Study the drawing (mm; zero at the part's minimum x, y, z) and answer. A direction names the side the tool comes from. Give positions to 0.01 mm unless a question says otherwise; leave off trailing zeros. Order: outer loops, then holes, each group sorted by start corner. A loop starts at its lowest first (then second) coordinate and runs counter-clockwise, first axis right, second up. Notation, with made-up numbers: (-32.5, -5.75) -> (24.5, -5.75) arc R16 cw to (24.5, 2.25) -> close; hole circle Ø11 at (23, 53.5). An arc over 180 degrees is marked (long way). Use a Markdown table: item, result. Add a question column.
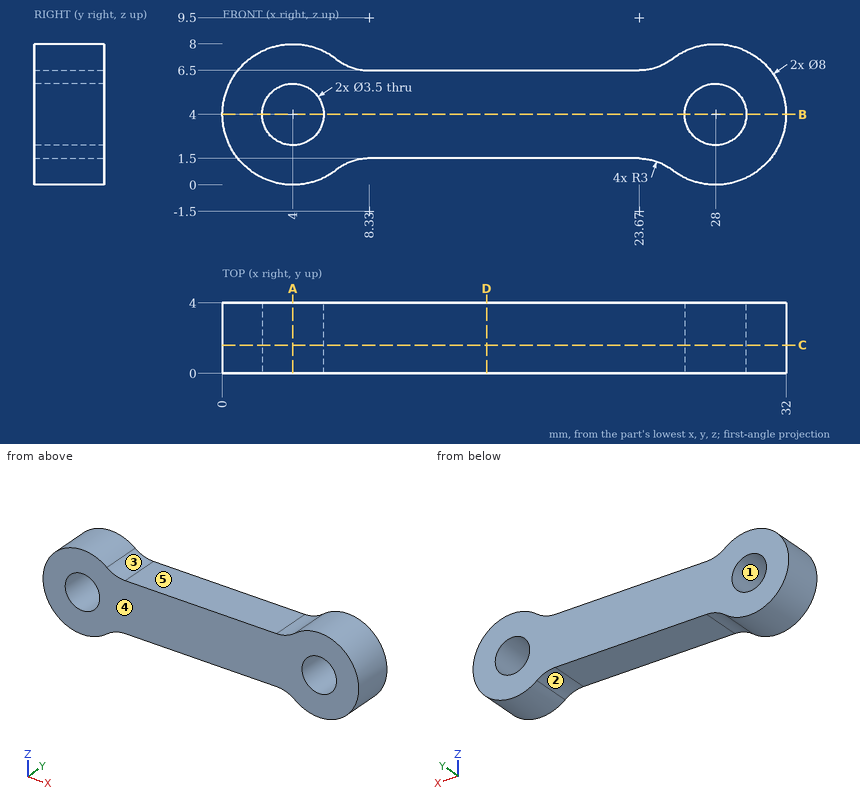
1) The part is cut by section A-A, the plane x = 4. Determine the outline of the cut face in (y, z).
2) Flat-ended cylindrical pins translate along their axes: pin 1 (2 mm diameter, centred on x = 16, y = 3, fed in from -Z); pin 2 (4.5 mm diameter, centred on x = 4, z = 4, fed in from +Y). Find the tip coordinate at first contact, or state that the pin passes through.
3) Which of the six approach directions +Z, -Z, +X, -X, +Y, -Y give full straight-line access (tool end or side, diameter ignored) to the marked faces 1, 2 and 3?
4) Determine the mould class of the marked faces 4 and 5 for opening direction X: released by +X, released by -X, zero draft, split by the parting line, or undercut.
5) The part is cut by section C-C, the plane y = 1.6. Determine the outline of the cut face in (x, z).
6) The part is cut by section B-B, the plane z = 4. Determine the outline of the cut face in (x, y), then the cut area to 3 significant figures.
7) Straight lines are drawn through the part: line 1 (X direction, y = 2, z = 4); line 2 (X direction, y = 3.4, z = 5); line 3 (Z direction, x = 4, y = 2.9). For each, find the intervals that lie inside material, in ascending order.
8) The part is cut by section D-D, the plane x = 15. Determine the outline of the cut face in (y, z), then the cut area to 3 significant figures.
A:
| question | item | result |
|---|---|---|
| 1 | outline | (0, 0) -> (4, 0) -> (4, 2.25) -> (0, 2.25) -> close; (0, 5.75) -> (4, 5.75) -> (4, 8) -> (0, 8) -> close |
| 2 | pin 1 | z = 1.5 |
| 2 | pin 2 | y = 4 |
| 3 | face 1 | +Y, -Y |
| 3 | face 2 | -Z, +Y, -Y |
| 3 | face 3 | +Z, +Y, -Y |
| 4 | face 4 | zero draft |
| 4 | face 5 | undercut |
| 5 | outline | (6.47, 0.86) arc R3 cw to (8.33, 1.5) -> (23.67, 1.5) arc R3 cw to (25.53, 0.86) arc R4 ccw (long way) to (25.53, 7.14) arc R3 cw to (23.67, 6.5) -> (8.33, 6.5) arc R3 cw to (6.47, 7.14) arc R4 ccw (long way) to start; hole circle Ø3.5 at (4, 4); hole circle Ø3.5 at (28, 4) |
| 6 | outline | (0, 0) -> (2.25, 0) -> (2.25, 4) -> (0, 4) -> close; (5.75, 0) -> (26.25, 0) -> (26.25, 4) -> (5.75, 4) -> close; (29.75, 0) -> (32, 0) -> (32, 4) -> (29.75, 4) -> close |
| 6 | area | 100 mm^2 |
| 7 | line 1 | 0 to 2.25, 5.75 to 26.25, 29.75 to 32 |
| 7 | line 2 | 0.13 to 2.56, 5.44 to 26.56, 29.44 to 31.87 |
| 7 | line 3 | 0 to 2.25, 5.75 to 8 |
| 8 | outline | (0, 1.5) -> (4, 1.5) -> (4, 6.5) -> (0, 6.5) -> close |
| 8 | area | 20.0 mm^2 |
